```python
from build123d import *

# Parameters (mm, degrees)
SKETCH_1_W      = 157
SKETCH_1_H      = 57
SKETCH_1_R      = 1.5
SKETCH_1_W_2    = 97
SKETCH_1_H_2    = 37
EXTRUDE_1_DEPTH = 4.5
SKETCH_2_W      = 3.5
SKETCH_2_H      = 30
SKETCH_2_W_2    = 50
SKETCH_2_H_2    = 3.5
EXTRUDE_2_DEPTH = 10


with BuildPart() as part:
    # 草图1 → 凸台-拉伸1 (new body)
    with BuildSketch(Plane.XY):
        Rectangle(SKETCH_1_W, SKETCH_1_H)
        with Locations((-65, 15)):
            Circle(SKETCH_1_R, mode=Mode.SUBTRACT)
        with Locations((65, 15)):
            Circle(SKETCH_1_R, mode=Mode.SUBTRACT)
        with Locations((-65, -15)):
            Circle(SKETCH_1_R, mode=Mode.SUBTRACT)
        with Locations((65, -15)):
            Circle(SKETCH_1_R, mode=Mode.SUBTRACT)
        Rectangle(SKETCH_1_W_2, SKETCH_1_H_2, mode=Mode.SUBTRACT)
    extrude(amount=EXTRUDE_1_DEPTH)

    # 草图2 → 凸台-拉伸2 (add)
    with BuildSketch(Plane.XY.offset(4.5)):
        with Locations((-76.75, 0)):
            Rectangle(SKETCH_2_W, SKETCH_2_H)
        with Locations((76.75, 0)):
            Rectangle(SKETCH_2_W, SKETCH_2_H)
        with Locations((0, 26.75)):
            Rectangle(SKETCH_2_W_2, SKETCH_2_H_2)
        with Locations((0, -26.75)):
            Rectangle(SKETCH_2_W_2, SKETCH_2_H_2)
    extrude(amount=EXTRUDE_2_DEPTH)


solid = part.part
```
Can you work these out from the model? Positions are in its coordinate system, mm. A direction names the side the tool comes from. Coordinates: 2 decimals unless noted, no trailing zeros. Order: outer loops, then holes, each group sorted by start corner. A loop starts at its lowest first (then second) coordinate and runs counter-clockwise, first axis right, second up. Notation, with made-up numbers: (67.25, -14) -> (86.25, -14) arc R9 ccw to (86.25, 0) -> close; hole circle Ø8 at (41, 56.25). An arc over 180 degrees is marked (long way). Write each question's results on one line, items separated by ' | '.
Item 1: I'm going to push flat-ended pins straight in: pin 1 Ø4 at (x, z) = (76, 9) entering from +Y; pin 2 Ø3.5 at (x, y) = (-65, 15) entering from +Z; pin 3 Ø1 at (y, z) = (-27.5, 11) entering from -X. Where does each tip first touch, or does it pass through?
Results are:
pin 1: y = 15 | pin 2: z = 4.5 | pin 3: x = -25
Item 2: I want a section at D-D, the plane z = 2. Write out the boundary of the cut face in (x, y), then the cut area to 3 significant figures.
Results are:
outline: (-78.5, -28.5) -> (78.5, -28.5) -> (78.5, 28.5) -> (-78.5, 28.5) -> close; hole circle Ø3 at (-65, -15); hole circle Ø3 at (-65, 15); hole (-48.5, -18.5) -> (48.5, -18.5) -> (48.5, 18.5) -> (-48.5, 18.5) -> close; hole circle Ø3 at (65, -15); hole circle Ø3 at (65, 15) | area: 5,330 mm²
Item 3: I want a section at B-B, the plane y = -6. Write out the boundary of the cut face in (x, z), then the cut area to 3 significant figures.
Results are:
outline: (-78.5, 0) -> (-48.5, 0) -> (-48.5, 4.5) -> (-75, 4.5) -> (-75, 14.5) -> (-78.5, 14.5) -> close; (48.5, 0) -> (78.5, 0) -> (78.5, 14.5) -> (75, 14.5) -> (75, 4.5) -> (48.5, 4.5) -> close | area: 340 mm²
Item 4: I want a section at A-A, the plane x = -20. Write out the boundary of the cut face in (y, z).
Results are:
outline: (-28.5, 0) -> (-18.5, 0) -> (-18.5, 4.5) -> (-25, 4.5) -> (-25, 14.5) -> (-28.5, 14.5) -> close; (18.5, 0) -> (28.5, 0) -> (28.5, 14.5) -> (25, 14.5) -> (25, 4.5) -> (18.5, 4.5) -> close
Item 5: If we mould it in two halves opening along X, with no side actions, what happens to faces 4 (the face through (-78.5, 0, 6)), 5 (the face through (-77, -15, 9)), 6 (the face through (75, 0, 9)), 7 (the face through (-63.57, -14.55, 2.22))? For each: +X half, -X half, draft (parallel to the pull), parting line (faces both ways), or undercut.
Results are:
face 4: -X half | face 5: draft | face 6: undercut | face 7: undercut
Item 6: I want a section at C-C, the plane x = 65. Write out the boundary of the cut face in (y, z).
Results are:
outline: (-28.5, 0) -> (-16.5, 0) -> (-16.5, 4.5) -> (-28.5, 4.5) -> close; (-13.5, 0) -> (13.5, 0) -> (13.5, 4.5) -> (-13.5, 4.5) -> close; (16.5, 0) -> (28.5, 0) -> (28.5, 4.5) -> (16.5, 4.5) -> close
Item 7: Which directions (+Z, -Z, +X, -X, +Y, -Y) give clear straight access to the entire face, cutting with the end or side of a thin tool? Please do faces 1 (the face through (48.5, 0, 2)), 2 (the face through (77, -15, 9)), 3 (the face through (0, 25, 9)).
Results are:
face 1: +Z, -Z | face 2: +Z, +X, -X, -Y | face 3: +Z, +X, -X
Item 8: If I drill on line 1 along Y through (x, z) = (-65, 2.9); line 2 along X through (y, z) = (10.5, 8.5); line 3 along Y through (x, z) = (-31.5, 2.5), over which ranges is the centre line in solid material (lowest first)?
Results are:
line 1: -28.5 to -16.5, -13.5 to 13.5, 16.5 to 28.5 | line 2: -78.5 to -75, 75 to 78.5 | line 3: -28.5 to -18.5, 18.5 to 28.5
